Build history of the part. All positions in model axes, mm. Give positions to 0.01 mm unless a question says otherwise; leave off trailing zeros. Write each loop counter-clockwise with the first axis right and the second up, starting at its lowest first coordinate (ties: lowest second). Pieces come first, ordered by that corner, then holes. Notation, with made-up numbers: (58, 54.5) -> (86, 54.5) arc R15 cw to (86, 79.5) -> close; hole circle Ø8 at (2, 35.5). An arc over 180 degrees is marked (long way). Put each result on its own line as item: value.
from build123d import *

# Parameters (mm, degrees)
SKETCH1_W           = 100
SKETCH1_H           = 20
BOSS_EXTRUDE1_DEPTH = 2
FILLET6_R           = 1
FILLET7_R           = 1
FILLET8_R           = 1
FILLET9_R           = 1
BOSS_EXTRUDE2_DEPTH = 1
BOSS_EXTRUDE3_START = 1
BOSS_EXTRUDE3_DEPTH = 1
SKETCH4_R           = 1.5
CUT_EXTRUDE4_DEPTH  = 11


with BuildPart() as part:
    # Sketch1 → Boss-Extrude1 (new body)
    with BuildSketch(Plane.XY):
        with Locations((4.951011889, -6.24877109)):
            Rectangle(SKETCH1_W, SKETCH1_H)
    extrude(amount=BOSS_EXTRUDE1_DEPTH)

    # Fillet6
    fillet6_edges = [part.edges().sort_by_distance(p)[0] for p in [
        (54.951011889, -16.24877109, 1),
    ]]
    fillet(fillet6_edges, radius=FILLET6_R)

    # Fillet7
    fillet7_edges = [part.edges().sort_by_distance(p)[0] for p in [
        (-45.048988111, -16.24877109, 1),
    ]]
    fillet(fillet7_edges, radius=FILLET7_R)

    # Fillet8
    fillet8_edges = [part.edges().sort_by_distance(p)[0] for p in [
        (-45.048988111, 3.75122891, 1),
    ]]
    fillet(fillet8_edges, radius=FILLET8_R)

    # Fillet9
    fillet9_edges = [part.edges().sort_by_distance(p)[0] for p in [
        (54.951011889, 3.75122891, 1),
    ]]
    fillet(fillet9_edges, radius=FILLET9_R)

    # Sketch2 → Boss-Extrude2 (add)
    with BuildSketch(Plane(origin=(0, -7.24877109, 0), x_dir=(-1, 0, 0), z_dir=(0, -1, 0))):
        with BuildLine():
            Line((-9.730976741, 0), (-9.730976741, 15))
            ThreePointArc((-9.730976741, 15), (-7.730976741, 17), (-5.730976741, 15))
            Line((-5.730976741, 15), (-5.730976741, 0))
            Line((-5.730976741, 0), (-9.730976741, 0))
        make_face()
    extrude(amount=BOSS_EXTRUDE2_DEPTH)

    # Sketch3 → Boss-Extrude3 (add)
    with BuildSketch(Plane(origin=(0, -5.24877109, 0), x_dir=(1, 0, 0), z_dir=(0, 1, 0)).offset(BOSS_EXTRUDE3_START)):
        with BuildLine():
            Line((5.730976741, 0), (5.730976741, 15))
            ThreePointArc((5.730976741, 15), (7.730976741, 17), (9.730976741, 15))
            Line((9.730976741, 15), (9.730976741, 0))
            Line((9.730976741, 0), (5.730976741, 0))
        make_face()
    extrude(amount=-BOSS_EXTRUDE3_DEPTH)

    # Sketch4 → Cut-Extrude4 (cut)
    with BuildSketch(Plane(origin=(0, -4.24877109, 0), x_dir=(1, 0, 0), z_dir=(0, 1, 0))):
        with Locations(Location((7.730976741, 15, 0), (0, 0, 270))):
            Circle(SKETCH4_R)
        with Locations(Location((7.730976741, 5, 0), (0, 0, 270))):
            Circle(SKETCH4_R)
    extrude(amount=-CUT_EXTRUDE4_DEPTH, mode=Mode.SUBTRACT)


solid = part.part
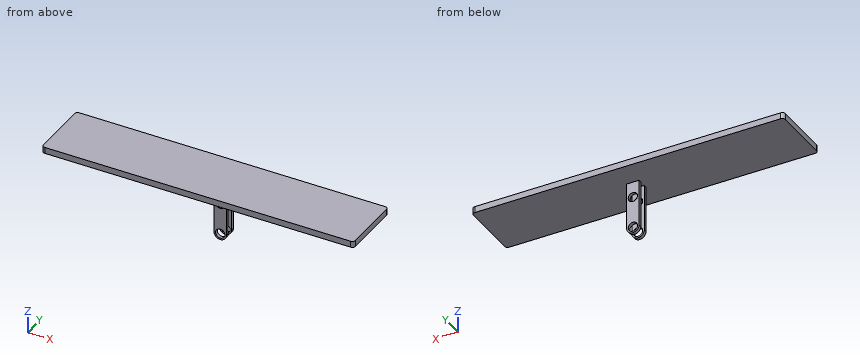
1) Pin check, flat tips, straight feed: pin 1 (0.8 mm diameter, centred on y = -4.5, z = -7.5, fed in from -X); pin 2 (3 mm diameter, centred on x = 8, z = -11.5, fed in from +Y); pin 3 (10 mm diameter, centred on x = -7.5, y = -4, fed in from -Z). Stop position of each tip, or through.
Filled sheet:
pin 1: x = 5.73
pin 2: y = -4.25
pin 3: z = 0
2) Wall check: L1, parallel to X at y = -7.5, z = -15; L2, parallel to Z at x = 2.5, y = -3; L3, parallel to X at y = -4.5, z = -8.25. Give the ranges that are in metal, low to high.
Filled sheet:
L1: 5.73 to 6.23, 9.23 to 9.73
L2: 0 to 2
L3: 5.73 to 9.73
3) Slice it at C-C (y = 1). Write the cut outline in (x, z).
Filled sheet:
outline: (-45.05, 0) -> (54.95, 0) -> (54.95, 2) -> (-45.05, 2) -> close
4) Slice it at B-B (z = -11.5). Write the cut outline in (x, y), plus the area to 3 significant figures.
Filled sheet:
outline: (5.73, -8.25) -> (9.73, -8.25) -> (9.73, -7.25) -> (5.73, -7.25) -> close; (5.73, -5.25) -> (9.73, -5.25) -> (9.73, -4.25) -> (5.73, -4.25) -> close
area: 8.00 mm2
5) Slice it at D-D (x = 31.5). Write the cut outline in (y, z).
Filled sheet:
outline: (-16.25, 0) -> (3.75, 0) -> (3.75, 2) -> (-16.25, 2) -> close
6) Slice it at A-A (z = -5). Write the cut outline in (x, y), plus the area to 3 significant figures.
Filled sheet:
outline: (5.73, -8.25) -> (6.23, -8.25) -> (6.23, -7.25) -> (5.73, -7.25) -> close; (5.73, -5.25) -> (6.23, -5.25) -> (6.23, -4.25) -> (5.73, -4.25) -> close; (9.23, -8.25) -> (9.73, -8.25) -> (9.73, -7.25) -> (9.23, -7.25) -> close; (9.23, -5.25) -> (9.73, -5.25) -> (9.73, -4.25) -> (9.23, -4.25) -> close
area: 2.00 mm2
